Build history of the part. All positions in model axes, mm. Face numbers are marked on the shaded views. A direction names the side the tool comes from. Round coordinates to 2 decimals unless told otherwise and drop trailing zeros. Loops run counter-clockwise (first coordinate to the right, second up) from the corner with the lowest first, then second, coordinate; pieces in that order, holes last.
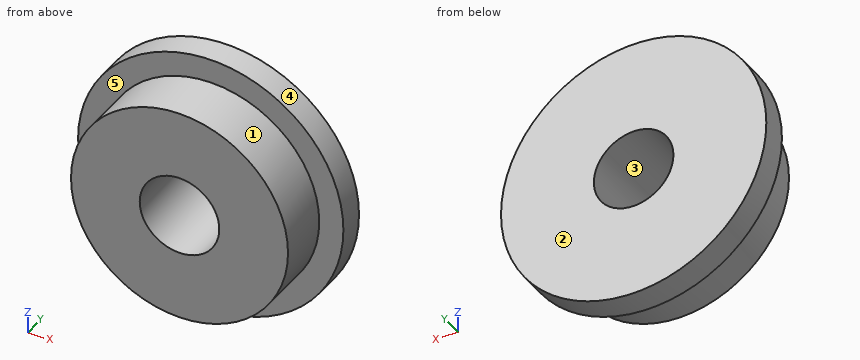
from build123d import *

# Parameters (mm, degrees)
F0_R     = 25.9715
F1_DEPTH = 12.7
F2_R     = 31.75
F3_DEPTH = 6.35
F4_R     = 9.525
F5_DEPTH = 19.05


with BuildPart() as f1:
    # F0 (on Front) → F1 (new body)
    with BuildSketch(Plane.XZ):
        Circle(F0_R)
    extrude(amount=F1_DEPTH)

    # F2 (on face) → F3 (join)
    with BuildSketch(Plane(origin=(0, 0, 0), x_dir=(-1, 0, 0), z_dir=(0, 1, 0))):
        Circle(F2_R)
    extrude(amount=F3_DEPTH)

    # F4 (on face) → F5 (cut, through all)
    with BuildSketch(Plane(origin=(0, 6.35, 0), x_dir=(-1, 0, 0), z_dir=(0, 1, 0))):
        Circle(F4_R)
    extrude(amount=-F5_DEPTH, mode=Mode.SUBTRACT)


solid = f1.part
(1) Which spindle directions (+Z, -Z, +X, -X, +Y, -Y) get a long thin tool onto all of the face, cutting with end or side? Do the marked faces 1 and 2. Say none if no direction does.
Responses:
face 1: -Y
face 2: +Z, -Z, +X, -X, +Y
(2) Pin check, flat tips, straight feed: P1, Ø5, axis at x = -14.5, y = -10, coming from the +Z side; P2, Ø2, axis at y = -6.5, z = 21, coming from the -X side; P3, Ø2, axis at x = -4, y = -9.5, coming from the -Z side. Stop position of each tip, or through.
Responses:
P1: stops at z = 23.03
P2: stops at x = -16.57
P3: stops at z = -25.8
(3) Probe line 1 (Z direction, x = 0, y = -0.5) (1 decimal); line 2 (Y direction, x = 28.5, z = -9.5); line 3 (X direction, y = 2.5, z = 2). List the from-to ranges inside material, lowest first.
Responses:
line 1: z = -26 to -9.5, 9.5 to 26
line 2: y = 0 to 6.35
line 3: x = -31.69 to -9.31, 9.31 to 31.69
(4) Slice it at D-D on z = -23. List the corners of the cut face in (x, y), plus the area to 3 significant figures.
Responses:
outline: (-21.89, 0) - (-12.06, 0) - (-12.06, -12.7) - (12.06, -12.7) - (12.06, 0) - (21.89, 0) - (21.89, 6.35) - (-21.89, 6.35) - close
area: 584 mm2
(5) Pull direction Z, two halves, no side cores. Call the marked faces 3, 4 and 5: +Z half, -Z half, draft (parallel to the pull), parting line (faces both ways), or undercut.
Responses:
face 3: undercut
face 4: parting line
face 5: draft
